```python
from build123d import *

# Parameters (mm, degrees)
SALIENTE_EXTRUIR1_DEPTH = 10
CROQUIS2_R              = 1.5
SALIENTE_EXTRUIR2_DEPTH = 6
CROQUIS3_R              = 1.5
CORTAR_EXTRUIR1_DEPTH   = 6


with BuildPart() as part:
    # Croquis1 → Saliente-Extruir1 (new body)
    with BuildSketch(Plane(origin=(0, 0, 0), x_dir=(1, 0, 0), z_dir=(0, 1, 0))):
        Polygon((0, 3.175426481), (-2.75, 1.58771324), (-2.75, -1.58771324), (0, -3.175426481), (2.75, -1.58771324), (2.75, 1.58771324), align=None)
    extrude(amount=SALIENTE_EXTRUIR1_DEPTH)

    # Croquis2 → Saliente-Extruir2 (add)
    with BuildSketch(Plane.XZ):
        Circle(CROQUIS2_R)
    extrude(amount=SALIENTE_EXTRUIR2_DEPTH)

    # Croquis3 → Cortar-Extruir1 (cut)
    with BuildSketch(Plane(origin=(0, 10, 0), x_dir=(1, 0, 0), z_dir=(0, 1, 0))):
        Circle(CROQUIS3_R)
    extrude(amount=-CORTAR_EXTRUIR1_DEPTH, mode=Mode.SUBTRACT)


solid = part.part
```
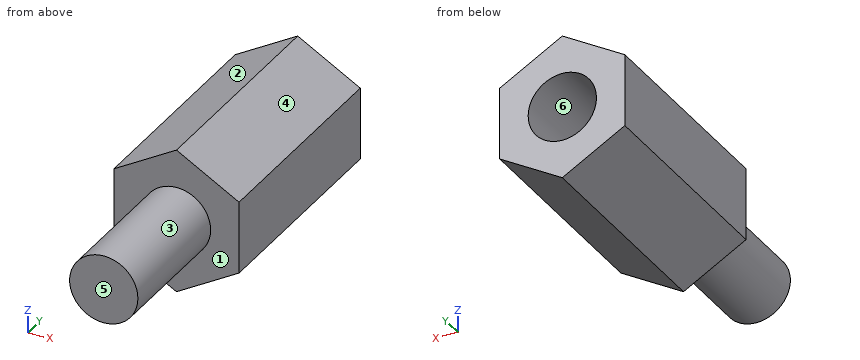
Verification items for the finished model (mm, model axes). Face numbers are marked on the shaded views. A direction names the side the tool comes from. Round coordinates to 2 decimals unless told otherwise and drop trailing zeros. Order: outer loops, then holes, each group sorted by start corner. A loop starts at its lowest first (then second) coordinate and runs counter-clockwise, first axis right, second up. Notation, with made-up numbers: (-33, -11) -> (10, -11) arc R33 ccw to (10, 21) -> close; hole circle Ø9 at (29.5, -12.5). An arc over 180 degrees is marked (long way). Put each result on its own line as item: value. Start each with the question number.
(1) Section check A-A (y = 6.25). Enter the section's corners in (x, z).
(2) Material ranges on line 1 along X through (y, z) = (7, 0); line 2 along Y through (x, z) = (-1.15, 0); line 3 along X through (y, z) = (9.5, -0.75), recorded low to high.
(3) Section check C-C (x = -0.5). Enter the section's corners in (y, z), then the cut area to 3 significant figures.
(4) Tool access check on the marked faces 1 and 2. Record the directions out of +Z, -Z, +X, -X, +Y, -Y that give a thin tool (end or side, any length) a straight path to the whole face; none if there is none.
(5) Depth check by flat-ended pin: pin 1 Ø0.9 at (x, z) = (0, 0) entering from +Y; pin 2 Ø3 at (x, y) = (-1.5, -1) entering from +Z; pin 3 Ø1 at (y, z) = (-1.5, -0.5) entering from -X. Enter the tip coordinate at first touch or a pass-through.
(6) Draft check along Z on the marked faces 3, 4, 5 and 6. Enter one of: +Z half, -Z half, draft (parallel to the pull), parting line (faces both ways), or undercut.
(7) Section check D-D (y = 0.5). Enter the section's corners in (x, z).
(8) Section check B-B (z = 0). Enter the section's corners in (x, y), then the cut area to 3 significant figures.
Completed:
1. outline: (-2.75, -1.59) -> (0, -3.18) -> (2.75, -1.59) -> (2.75, 1.59) -> (0, 3.18) -> (-2.75, 1.59) -> close; hole circle Ø3 at (0, 0)
2. line 1: x = -2.75 to -1.5, 1.5 to 2.75
2. line 2: y = -6 to 4
2. line 3: x = -2.75 to -1.3, 1.3 to 2.75
3. outline: (-6, -1.41) -> (0, -1.41) -> (0, -2.89) -> (10, -2.89) -> (10, -1.41) -> (4, -1.41) -> (4, 1.41) -> (10, 1.41) -> (10, 2.89) -> (0, 2.89) -> (0, 1.41) -> (-6, 1.41) -> close
3. area: 57.7 mm2
4. face 1: -Y
4. face 2: +Z, -X, +Y, -Y
5. pin 1: stops at y = 4
5. pin 2: stops at z = 2.95
5. pin 3: stops at x = -1.5
6. face 3: parting line
6. face 4: +Z half
6. face 5: draft
6. face 6: undercut
7. outline: (-2.75, -1.59) -> (0, -3.18) -> (2.75, -1.59) -> (2.75, 1.59) -> (0, 3.18) -> (-2.75, 1.59) -> close
8. outline: (-2.75, 0) -> (-1.5, 0) -> (-1.5, -6) -> (1.5, -6) -> (1.5, 0) -> (2.75, 0) -> (2.75, 10) -> (1.5, 10) -> (1.5, 4) -> (-1.5, 4) -> (-1.5, 10) -> (-2.75, 10) -> close
8. area: 55.0 mm2
